Read the model definition and answer for the solid it produces. Units are mm, in the model's axes. Give positions to 0.01 mm unless a question says otherwise; leave off trailing zeros. Loops run counter-clockwise (first coordinate to the right, second up) from the corner with the lowest first, then second, coordinate; pieces in that order, holes last. Notation, with made-up numbers: (37, 66.5) - (69, 66.5) arc R20 ccw to (69, 79.5) - close; hole circle Ø9 at (-30, 37.25). An arc over 180 degrees is marked (long way). Use a Markdown table: item, result. Add a question column.
Item 1: A cutting plane is placed at D-D (z = -117.5). Determine the outline of the cut face in (x, y), plus the area to 3 significant figures.
Item 2: Each of these flat-tipped pins is pushed along its axis until it touches: P1, Ø12, axis at y = -355.5, z = 58, coming from the +X side; P2, Ø2, axis at x = 89.5, y = 113, coming from the -Z side; P3, Ø2, axis at x = -24.5, y = -66, coming from the +Z side. Where does it stop, or does it pass through?
Item 3: Consider probe 1 along X at (y, z) = (-228, -198.5); probe 2 along X at (y, z) = (-197, -94.5); probe 3 along Z at (x, y) = (-75, -286). Determine where each line is inside the solid, lowest interval first. Write a range as [from, to].
Item 4: A cutting plane is placed at A-A (z = 0). Determine the outline of the cut face in (x, y).
Item 5: A cutting plane is placed at B-B (x = 191.5). Determine the outline of the cut face in (y, z).
from build123d import *

# Parameters (mm, degrees)
F0_R     = 254
F0_R_2   = 244.5
F1_DEPTH = 457.5
F3_DEPTH = 375


with BuildPart() as f1:
    # F0 (on Front) → F1 (new body, symmetric)
    with BuildSketch(Plane.XZ):
        Circle(F0_R)
        Circle(F0_R_2, mode=Mode.SUBTRACT)
    extrude(amount=F1_DEPTH, both=True)

    # F2 (on Front) → F3 (cut, symmetric)
    with BuildSketch(Plane.XZ):
        with BuildLine():
            ThreePointArc((237.1294283303, -91.0254591845), (209.32805191, 143.8671841789), (0, 254))
            Line((0, 254), (0, 244.5))
            ThreePointArc((0, 244.5), (201.4988531181, 138.4863249281), (228.2604142786, -87.6209636638))
            Line((228.2604142786, -87.6209636638), (237.1294283303, -91.0254591845))
        make_face()
        with BuildLine():
            ThreePointArc((228.2604142786, -87.6209636638), (201.4988531181, 138.4863249281), (0, 244.5))
            Line((0, 244.5), (0, 0))
            Line((0, 0), (228.2604142786, -87.6209636638))
        make_face()
    extrude(amount=F3_DEPTH, both=True, mode=Mode.SUBTRACT)


solid = f1.part
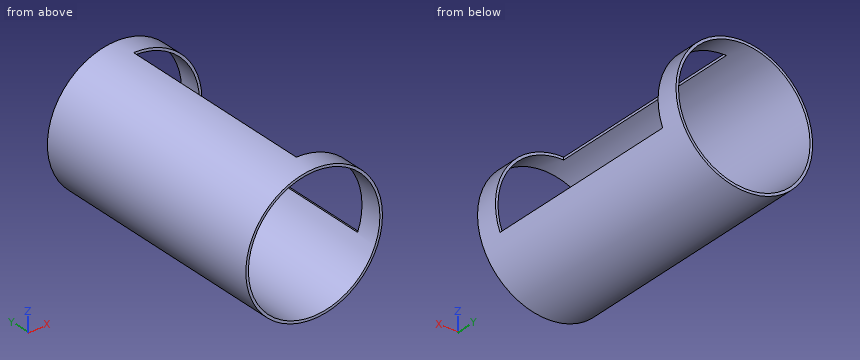
Geometry says:
| question | item | result |
|---|---|---|
| 1 | outline | (-225.19, -457.5) - (-214.42, -457.5) - (-214.42, 457.5) - (-225.19, 457.5) - close; (214.42, -457.5) - (225.19, -457.5) - (225.19, 457.5) - (214.42, 457.5) - close |
| 1 | area | 19,700 mm² |
| 2 | P1 | x = -235.98 |
| 2 | P2 | z = -238.08 |
| 2 | P3 | z = 252.91 |
| 3 | probe 1 | [-158.47, -142.75], [142.75, 158.47] |
| 3 | probe 2 | [-235.77, -225.5], [225.5, 235.77] |
| 3 | probe 3 | [-242.67, -232.71], [232.71, 242.67] |
| 4 | outline | (-254, -457.5) - (-244.5, -457.5) - (-244.5, 457.5) - (-254, 457.5) - close; (244.5, -457.5) - (254, -457.5) - (254, -375) - (244.5, -375) - close; (244.5, 375) - (254, 375) - (254, 457.5) - (244.5, 457.5) - close |
| 5 | outline | (-457.5, -166.86) - (457.5, -166.86) - (457.5, -152.01) - (-457.5, -152.01) - close; (-457.5, 152.01) - (-375, 152.01) - (-375, 166.86) - (-457.5, 166.86) - close; (375, 152.01) - (457.5, 152.01) - (457.5, 166.86) - (375, 166.86) - close |
